Read the model definition and answer for the solid it produces. Units are mm, in the model's axes. Coordinates: 2 decimals unless noted, no trailing zeros. Write each loop counter-clockwise with the first axis right and the second up, starting at its lowest first coordinate (ties: lowest second). Pieces come first, ordered by that corner, then holes.
Item 1: Section D-D (x = 40) is taken. Give the vertices of the cut face in (y, z).
Item 2: Section C-C (z = 79.5) is taken. Give the vertices of the cut face in (x, y), then the cut area to 3 significant figures.
Item 3: Section A-A (x = -17) is taken. Give the vertices of the cut face in (y, z).
Item 4: Section B-B (z = 19.5) is taken. Give the vertices of the cut face in (x, y), then the cut area to 3 significant figures.
Item 5: Each of these flat-tipped pins is pushed along its axis until it touches: P1, Ø1.5, axis at x = -67.5, y = -1, coming from the +Z side; P2, Ø1.5, axis at y = -1, z = 7, coming from the +X side; P3, Ø1.5, axis at y = -1.5, z = 1.5, coming from the -X side. Where does it stop, or does it pass through?
Item 6: Straight lines are drawn through the part: probe 1 along X at (y, z) = (-0.9, 8); probe 2 along X at (y, z) = (-2.8, 16); probe 3 along X at (y, z) = (-1.95, -41). For each, find the intervals that lie inside material, in ascending order.
from build123d import *

# Parameters (mm, degrees)
F0_R     = 10
F0_W     = 30
F0_H     = 8
F1_DEPTH = 3
F2_DEPTH = 3
F0_W_2   = 12.0982
F0_H_2   = 1.102668
F3_DEPTH = 3


with BuildPart() as f1:
    # F0 (on Front) → F1 (new body)
    with BuildSketch(Plane.XZ):
        Polygon((0, 89.465775), (-73.68011, 52.592348), (-3.317016, 52.592348), (4.682984, 52.592348), (74.850552, 52.592348), align=None)
        Polygon((9.737339, 75.563721), (4.86867, 67.130938), (-4.86867, 67.130938), (-9.737339, 75.563721), (-4.86867, 83.996505), (4.86867, 83.996505), align=None, mode=Mode.SUBTRACT)
        Polygon((-73.68011, 52.592348), (-73.582347, 26.296174), (-72.12289, 26.290895), (-59.835819, 26.246452), (-3.317016, 26.042022), (-3.317016, 52.592348), align=None)
        with Locations((-41.317016, 39.155915)):
            Circle(F0_R, mode=Mode.SUBTRACT)
        Polygon((74.850552, 52.592348), (4.682984, 52.592348), (4.682984, 26.013086), (61.834292, 25.806368), (72.453672, 25.767957), (74.753497, 25.759638), align=None)
        with Locations((42.65259, 38.629778)):
            Circle(F0_R, mode=Mode.SUBTRACT)
        Polygon((4.682984, 26.013086), (4.682984, 0), (61.930233, 0), (61.834292, 25.806368), align=None)
        Polygon((42.682735, 3.071828), (12.682931, 3.180338), (12.682931, 11.180175), (42.65259, 11.180175), align=None, mode=Mode.SUBTRACT)
        Polygon((-59.835819, 26.246452), (-59.738242, 0), (-3.317016, 0), (-3.317016, 26.042022), align=None)
        Polygon((-11.317016, 11.180175), (-11.317016, 3.180338), (-41.31682, 3.288848), (-41.346562, 11.288793), align=None, mode=Mode.SUBTRACT)
        Polygon((-73.484585, 0), (-73.484585, -25.583768), (-71.836442, -25.577641), (-59.738242, -25.532663), (-3.317016, -25.322903), (-3.317016, 0), (-59.738242, 0), (-72.12289, 0), align=None)
        with Locations((-41.317016, -11.177788)):
            Circle(F0_R, mode=Mode.SUBTRACT)
        Polygon((4.682984, 0), (4.682984, -25.293161), (61.930233, -25.08033), (72.305258, -25.041758), (74.753389, -25.032656), (74.660324, 0), (72.549471, 0), (61.930233, 0), align=None)
        with Locations((42.682735, -12.054683)):
            Circle(F0_R, mode=Mode.SUBTRACT)
        Polygon((-59.738242, -50.064869), (-59.738242, -51.167537), (-3.317016, -51.167537), (-3.317016, -40.167537), (4.682984, -40.167537), (4.682984, -51.167537), (61.835875, -51.167537), (61.839649, -50.124135), (61.930233, -25.08033), (4.682984, -25.293161), (-3.317016, -25.322903), (-59.738242, -25.532663), align=None)
        with Locations((-26.317016, -44.189357)):
            Rectangle(F0_W, F0_H, mode=Mode.SUBTRACT)
        Polygon((12.682931, -48.311945), (12.682931, -40.311945), (42.682735, -40.420455), (42.682931, -48.311945), align=None, mode=Mode.SUBTRACT)
    extrude(amount=F1_DEPTH)

    # F0 (on Front) → F2 (join)
    with BuildSketch(Plane.XZ):
        Polygon((-73.582347, 26.296174), (-73.484585, 0), (-72.12289, 0), (-72.12289, 26.290895), align=None)
        Polygon((-73.484585, -25.583768), (-73.484585, -51.167537), (-71.836442, -51.167537), (-71.836442, -50.064869), (-71.836442, -25.577641), align=None)
        Polygon((74.660324, 0), (74.753497, 25.759638), (72.453672, 25.767957), (72.549471, 0), align=None)
        Polygon((72.398508, -50.124135), (72.402387, -51.167537), (74.850552, -51.167537), (74.753389, -25.032656), (72.305258, -25.041758), align=None)
    extrude(amount=F2_DEPTH)

    # F0 (on Front) → F3 (join)
    with BuildSketch(Plane.XZ):
        Polygon((61.839649, -50.124135), (61.835875, -51.167537), (72.402387, -51.167537), (72.398508, -50.124135), align=None)
        with Locations((-65.787342, -50.616203)):
            Rectangle(F0_W_2, F0_H_2)
    extrude(amount=F3_DEPTH)


solid = f1.part
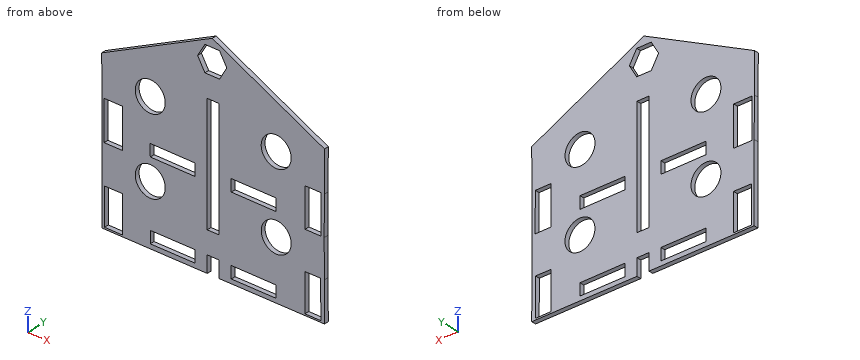
Established:
1. outline: (-3, -51.17) - (0, -51.17) - (0, -48.31) - (-3, -48.31) - close; (-3, -40.41) - (0, -40.41) - (0, -21.69) - (-3, -21.69) - close; (-3, -2.42) - (0, -2.42) - (0, 3.08) - (-3, 3.08) - close; (-3, 11.18) - (0, 11.18) - (0, 28.99) - (-3, 28.99) - close; (-3, 48.27) - (0, 48.27) - (0, 69.76) - (-3, 69.76) - close
2. outline: (-19.91, -3) - (-7.46, -3) - (-7.46, 0) - (-19.91, 0) - close; (7.46, -3) - (20.23, -3) - (20.23, 0) - (7.46, 0) - close
2. area: 75.6 mm2
3. outline: (-3, -51.17) - (0, -51.17) - (0, -48.19) - (-3, -48.19) - close; (-3, -40.19) - (0, -40.19) - (0, 3.2) - (-3, 3.2) - close; (-3, 11.2) - (0, 11.2) - (0, 80.96) - (-3, 80.96) - close
4. outline: (-73.56, -3) - (-72.12, -3) - (-72.12, 0) - (-73.56, 0) - close; (-59.81, -3) - (-3.32, -3) - (-3.32, 0) - (-59.81, 0) - close; (4.68, -3) - (61.86, -3) - (61.86, 0) - (4.68, 0) - close; (72.48, -3) - (74.73, -3) - (74.73, 0) - (72.48, 0) - close
4. area: 352 mm2
5. P1: stops at z = 56.06
5. P2: stops at x = 74.69
5. P3: stops at x = -73.49
6. probe 1: x = -73.51 to -72.12, -59.77 to -41.33, -11.32 to -3.32, 4.68 to 12.68, 42.66 to 61.9, 72.52 to 74.69
6. probe 2: x = -73.54 to -72.12, -59.8 to -3.32, 4.68 to 61.87, 72.49 to 74.72
6. probe 3: x = -73.48 to -71.84, -59.74 to -41.32, -11.32 to -3.32, 4.68 to 12.68, 42.68 to 61.87, 72.36 to 74.81
